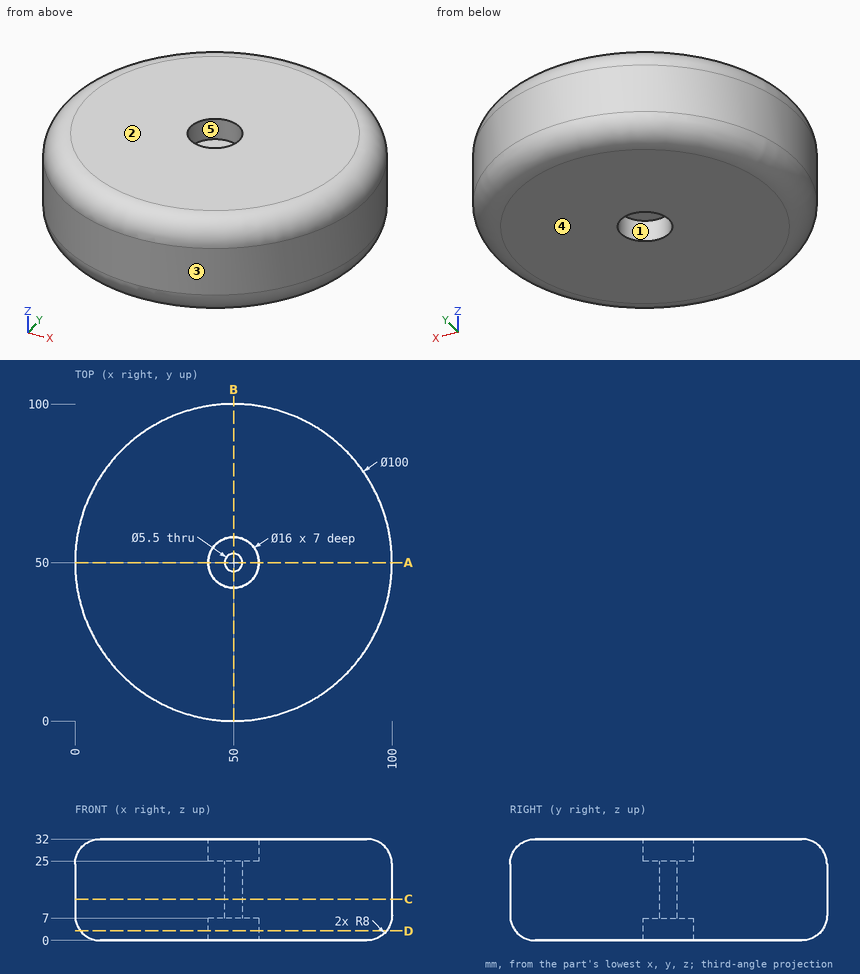
Drawing for the job (mm, zero at the part's lowest x, y, z). A direction names the side the tool comes from. Give positions to 0.01 mm unless a question says otherwise; leave off trailing zeros. Order: outer loops, then holes, each group sorted by start corner. A loop starts at its lowest first (then second) coordinate and runs counter-clockwise, first axis right, second up. Notation, with made-up numbers: M 21.25,-5.5 L 80.25,-5.5 A13 ccw 80.25,4.5 Z; hole C 52.5,3 d4. An arc over 180 degrees is marked long. Use a Markdown table: item, result. Add a question column.
(1) Probe line 1 along Y through (x, z) = (50, 17); line 2 along X through (y, z) = (45.5, 30.5); line 3 along Z through (x, y) = (61.5, 91). List the from-to ranges inside material, lowest first. Write a range as [from, to].
(2) Saw through at A-A, the plane y = 50. Give the cut face in (x, z).
(3) Mould opens along Y. For the marked faces 3, 4 and 5 say: +Y half, -Y half, draft (parallel to the pull), parting line (faces both ways), or undercut.
(4) Drop flat-ended pins along their axis: P1, Ø5, axis at x = 50, y = 53, coming from the -Z side; P2, Ø8, axis at x = 31, z = 17, coming from the +Y side; P3, Ø6, axis at x = 14, y = 54, coming from the -Z side; P4, Ø1.5, axis at x = 63, z = 13.5, coming from the +Y side. Give the stop position or say it passes through.
(5) 3-axis set-ups, long thin cutter, end or side, ignore diameter. For the marked faces 1 and 2: which of +Z, -Z, +X, -X, +Y, -Y reach the whole face in a straight line?
(6) Saw through at C-C, the plane z = 13. Give the cut face in (x, y).
(7) Saw through at D-D, the plane z = 3. Give the cut face in (x, y) (3 decimals), and give its area (3 significant figures).
Answer key:
| question | item | result |
|---|---|---|
| 1 | line 1 | [0, 47.25], [52.75, 100] |
| 1 | line 2 | [3.55, 43.39], [56.61, 96.45] |
| 1 | line 3 | [0.02, 31.98] |
| 2 | outline | M 0,8 A8 ccw 8,0 L 42,0 L 42,7 L 47.25,7 L 47.25,25 L 42,25 L 42,32 L 8,32 A8 ccw 0,24 Z; M 52.75,7 L 58,7 L 58,0 L 92,0 A8 ccw 100,8 L 100,24 A8 ccw 92,32 L 58,32 L 58,25 L 52.75,25 Z |
| 3 | face 3 | parting line |
| 3 | face 4 | draft |
| 3 | face 5 | undercut |
| 4 | P1 | z = 7 |
| 4 | P2 | y = 97.7 |
| 4 | P3 | z = 0 |
| 4 | P4 | y = 98.48 |
| 5 | face 1 | -Z |
| 5 | face 2 | +Z, +X, -X, +Y, -Y |
| 6 | outline | C 50,50 d100; hole C 50,50 d5.5 |
| 7 | outline | C 50,50 d96.49; hole C 50,50 d16 |
| 7 | area | 7,110 mm^2 |
